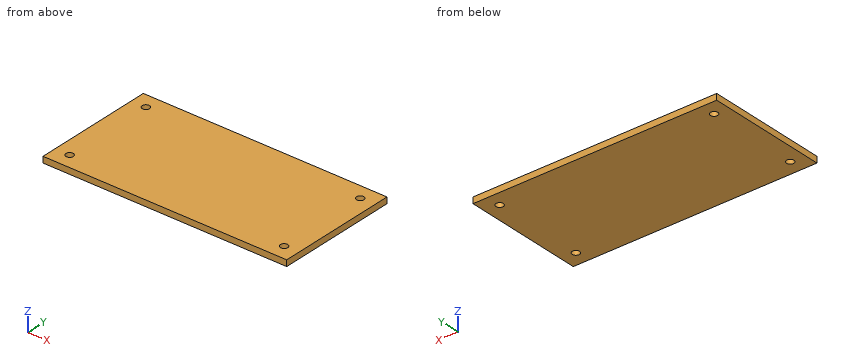
```python
from build123d import *

# Parameters (mm, degrees)
SKETCH_1_W          = 2000
SKETCH_1_H          = 1000
EXTRUDE_1_DEPTH     = 50
SKETCH_2_R          = 30
CUT_EXTRUDE_1_DEPTH = 1120.15146428
SKETCH_3_R          = 30
CUT_EXTRUDE_2_DEPTH = 1120.15146428
SKETCH_4_R          = 30
CUT_EXTRUDE_3_DEPTH = 1120.15146428
SKETCH_5_R          = 30
CUT_EXTRUDE_4_DEPTH = 1120.15146428


with BuildPart() as part:
    # 草图1 → 凸台-拉伸1 (new body)
    with BuildSketch(Plane.XY):
        Rectangle(SKETCH_1_W, SKETCH_1_H)
    extrude(amount=EXTRUDE_1_DEPTH)

    # 草图2 → 切除-拉伸1 (cut, through all)
    with BuildSketch(Plane.XY):
        with Locations((880, 380)):
            Circle(SKETCH_2_R)
    extrude(amount=CUT_EXTRUDE_1_DEPTH, mode=Mode.SUBTRACT)

    # 草图3 → 切除-拉伸2 (cut, through all)
    with BuildSketch(Plane.XY):
        with Locations((880, -380)):
            Circle(SKETCH_3_R)
    extrude(amount=CUT_EXTRUDE_2_DEPTH, mode=Mode.SUBTRACT)

    # 草图4 → 切除-拉伸3 (cut, through all)
    with BuildSketch(Plane.XY):
        with Locations((-880, 380)):
            Circle(SKETCH_4_R)
    extrude(amount=CUT_EXTRUDE_3_DEPTH, mode=Mode.SUBTRACT)

    # 草图5 → 切除-拉伸4 (cut, through all)
    with BuildSketch(Plane.XY):
        with Locations((-880, -380)):
            Circle(SKETCH_5_R)
    extrude(amount=CUT_EXTRUDE_4_DEPTH, mode=Mode.SUBTRACT)


solid = part.part
```
Part model, mm, in its own coordinate system. Round coordinates to 2 decimals unless told otherwise and drop trailing zeros. Order: outer loops, then holes, each group sorted by start corner. A loop starts at its lowest first (then second) coordinate and runs counter-clockwise, first axis right, second up. Notation, with made-up numbers: M 75.5,-36 L 133.5,-36 A12 cw 133.5,-13 Z; hole C 88.25,-14 d10. An arc over 180 degrees is marked long. Answer in a Markdown table with one row per item. Add a question column.
Q1. Cut at B-B on x = 880. Give the cut face in (y, z).
Q2. Wall check: L1, parallel to X at y = 380, z = 12.5; L2, parallel to Y at x = -880, z = 32.5. Give the ranges that are in metal, low to high. Write a range as from..to.
Q3. Cut at A-A on y = -380. Give the cut face in (x, z), and give its area (3 significant figures).
Established:
| question | item | result |
|---|---|---|
| 1 | outline | M -500,0 L -410,0 L -410,50 L -500,50 Z; M -350,0 L 350,0 L 350,50 L -350,50 Z; M 410,0 L 500,0 L 500,50 L 410,50 Z |
| 2 | L1 | x = -1000..-910, -850..850, 910..1000 |
| 2 | L2 | y = -500..-410, -350..350, 410..500 |
| 3 | outline | M -1000,0 L -910,0 L -910,50 L -1000,50 Z; M -850,0 L 850,0 L 850,50 L -850,50 Z; M 910,0 L 1000,0 L 1000,50 L 910,50 Z |
| 3 | area | 94,000 mm2 |
